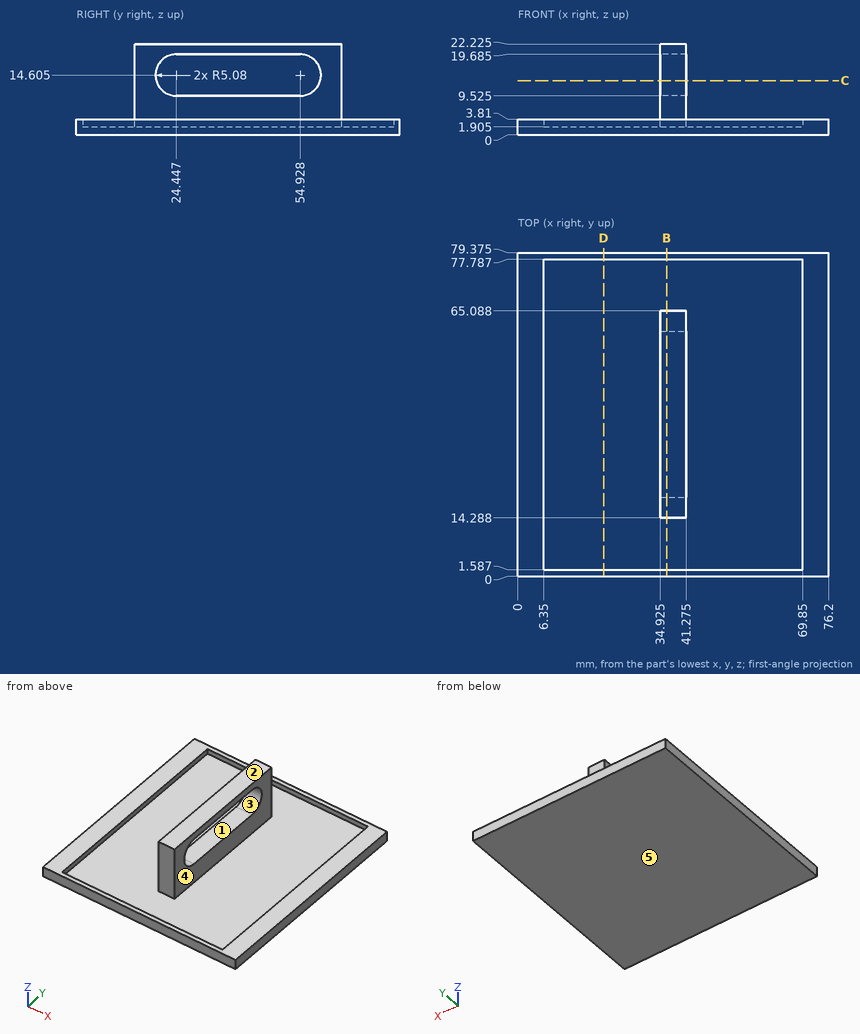
Can you work these out from the drawing? Everything is in mm from the part's minimum corner. A direction names the side the tool comes from. Coordinates: 2 decimals unless noted, no trailing zeros. Loops run counter-clockwise (first coordinate to the right, second up) from the corner with the lowest first, then second, coordinate; pieces in that order, holes last. Notation, with made-up numbers: (41.25, -0.75) - (64.25, -0.75) arc R19 ccw to (64.25, 11.25) - close; hole circle Ø10 at (-10, 15.5). An arc over 180 degrees is marked (long way). Put each result on its own line as item: value. Start each with the question number.
Item 1: For pin 1 (5 mm diameter, centred on x = 37.5, z = 9, fed in from -Y); pin 2 (5 mm diameter, centred on x = 38, z = 15.5, fed in from +Y); pin 3 (6 mm diameter, centred on y = 49.5, z = 10, fed in from +X) (1 decimal); pin 4 (1 mm diameter, centred on y = 30.5, z = 18, fed in from +X), each with a flat end and sliding along its axis, tell me the tip position at first contact or that it passes through.
Item 2: Suppose I cut it at B-B (x = 36.5). Please give me the cut outline in (y, z) (1 decimal).
Item 3: If I drill on line 1 along X through (y, z) = (4, 3); line 2 along Z through (x, y) = (48, 55.5) (1 decimal); line 3 along Y through (x, z) = (65, 3) (1 decimal), over which ranges is the centre line in solid material (lowest first)?
Item 4: Which directions (+Z, -Z, +X, -X, +Y, -Y) give clear straight access to the entire face, cutting with the end or side of a thin tool? Please do the marked faces 1 and 2.
Item 5: If we mould it in two halves opening along Z, with no side actions, what happens to the marked faces 3, 4 and 5? For each: +Z half, -Z half, draft (parallel to the pull), parting line (faces both ways), or undercut.
Item 6: Suppose I cut it at D-D (x = 21). Please give me the cut outline in (y, z) (1 decimal).
Item 7: Suppose I cut it at C-C (z = 13.25). Please give me the cut outline in (x, y) (1 decimal).
Here are the results:
1. pin 1: y = 14.29
1. pin 2: y = 65.09
1. pin 3: x = 41.3
1. pin 4: through
2. outline: (0, 0) - (79.4, 0) - (79.4, 3.8) - (77.8, 3.8) - (77.8, 1.9) - (65.1, 1.9) - (65.1, 22.2) - (14.3, 22.2) - (14.3, 1.9) - (1.6, 1.9) - (1.6, 3.8) - (0, 3.8) - close; hole (24.4, 9.5) - (54.9, 9.5) arc R5.1 ccw to (54.9, 19.7) - (24.4, 19.7) arc R5.1 ccw to start
3. line 1: 0 to 6.35, 69.85 to 76.2
3. line 2: 0 to 1.9
3. line 3: 0 to 1.6, 77.8 to 79.4
4. face 1: +X, -X
4. face 2: +Z, +X, -X, +Y, -Y
5. face 3: undercut
5. face 4: draft
5. face 5: -Z half
6. outline: (0, 0) - (79.4, 0) - (79.4, 3.8) - (77.8, 3.8) - (77.8, 1.9) - (1.6, 1.9) - (1.6, 3.8) - (0, 3.8) - close
7. outline: (34.9, 14.3) - (41.3, 14.3) - (41.3, 19.6) - (34.9, 19.6) - close; (34.9, 59.8) - (41.3, 59.8) - (41.3, 65.1) - (34.9, 65.1) - close
